Geometry check sheet. Reference: the model listing, model coordinates, mm. Round coordinates to 2 decimals unless told otherwise and drop trailing zeros. Write each loop counter-clockwise with the first axis right and the second up, starting at its lowest first coordinate (ties: lowest second). Pieces come first, ordered by that corner, then holes.
Item 1: Cross-section at D-D (y = 65). Enter the section's corners in (x, z).
Item 2: Cross-section at C-C (x = 42). Enter the section's corners in (y, z).
Item 3: Scan lines: probe 1 along Y at (x, z) = (42, 1); probe 2 along Y at (x, z) = (25, 0.25); probe 3 along Y at (x, z) = (-7, 0.55). Record each from-to range of solid material in increasing order.
Item 4: Depth check by flat-ended pin: P1, Ø1, axis at y = 51.5, z = 0.5, coming from the +X side; P2, Ø1, axis at y = -53.5, z = 1, coming from the -X side. Enter the tip coordinate at first touch or a pass-through.
Item 5: Cross-section at B-B (z = 0.95). Enter the section's corners in (x, y).
Item 6: Cross-section at A-A (y = 7.5). Enter the section's corners in (x, z), then the cut area to 3 significant figures.
from build123d import *

# Parameters (mm, degrees)
CYLINDER002_R     = 25
CYLINDER002_DEPTH = 2
CYLINDER001_R     = 25
CYLINDER001_DEPTH = 2
BOX_W             = 90
BOX_H             = 7
BOX_DEPTH         = 2
CYLINDER_R        = 100
CYLINDER_DEPTH    = 2


with BuildPart() as cylinder002:
    # Cylinder002 → Cylinder002 (new body)
    with BuildSketch(Plane(origin=(42, 26.3, 0), x_dir=(1, 0, 0), z_dir=(0, 0, 1))):
        Circle(CYLINDER002_R)
    extrude(amount=CYLINDER002_DEPTH)


with BuildPart() as cylinder001:
    # Cylinder001 → Cylinder001 (new body)
    with BuildSketch(Plane(origin=(-45, 26.3, 0), x_dir=(1, 0, 0), z_dir=(0, 0, 1))):
        Circle(CYLINDER001_R)
    extrude(amount=CYLINDER001_DEPTH)


with BuildPart() as cube:
    # Box → Box (new body)
    with BuildSketch(Plane(origin=(-44, -56, 0), x_dir=(1, 0, 0), z_dir=(0, 0, 1))):
        with Locations((45, 3.5)):
            Rectangle(BOX_W, BOX_H)
    extrude(amount=BOX_DEPTH)


with BuildPart() as cut002:
    # Cylinder → Cylinder (new body)
    with BuildSketch(Plane.XY):
        Circle(CYLINDER_R)
    extrude(amount=CYLINDER_DEPTH)

    # Cut: cut Cube
    add(cube.part, mode=Mode.SUBTRACT)

    # Cut001: cut Cylinder001
    add(cylinder001.part, mode=Mode.SUBTRACT)

    # Cut002: cut Cylinder002
    add(cylinder002.part, mode=Mode.SUBTRACT)


solid = cut002.part
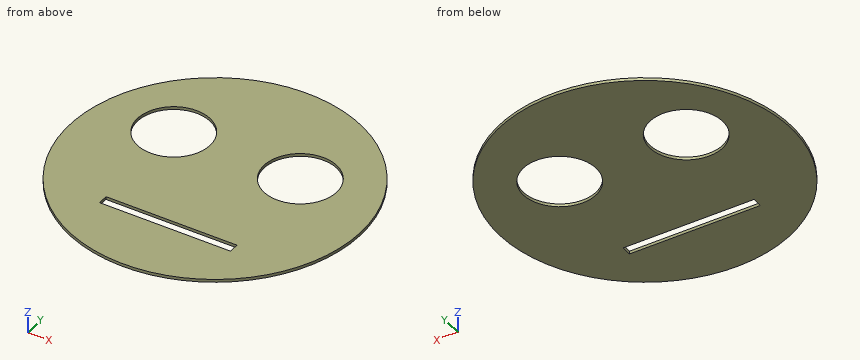
Resolved:
1. outline: (-75.99, 0) - (75.99, 0) - (75.99, 2) - (-75.99, 2) - close
2. outline: (-90.75, 0) - (-56, 0) - (-56, 2) - (-90.75, 2) - close; (-49, 0) - (1.3, 0) - (1.3, 2) - (-49, 2) - close; (51.3, 0) - (90.75, 0) - (90.75, 2) - (51.3, 2) - close
3. probe 1: y = -90.75 to -56, -49 to 1.3, 51.3 to 90.75
3. probe 2: y = -96.82 to -56, -49 to 7.97, 44.63 to 96.82
3. probe 3: y = -99.75 to -56, -49 to 99.75
4. P1: stops at x = 86.02
4. P2: stops at x = -84.8
5. outline: circle Ø200 at (0, 0); hole circle Ø50 at (-45, 26.3); hole (-44, -56) - (46, -56) - (46, -49) - (-44, -49) - close; hole circle Ø50 at (42, 26.3)
6. outline: (-99.72, 0) - (-61.48, 0) - (-61.48, 2) - (-99.72, 2) - close; (-28.52, 0) - (25.52, 0) - (25.52, 2) - (-28.52, 2) - close; (58.48, 0) - (99.72, 0) - (99.72, 2) - (58.48, 2) - close
6. area: 267 mm2
